CAD build for the part. Positions are in the model's coordinates, mm. Face numbers are marked on the shaded views. A direction names the side the tool comes from. Round coordinates to 2 decimals unless told otherwise and drop trailing zeros. Loops run counter-clockwise (first coordinate to the right, second up) from the corner with the lowest first, then second, coordinate; pieces in that order, holes last. Notation, with made-up numbers: M -26.75,55.5 L 27.25,55.5 A16 cw 27.25,76.5 Z; hole C 22.25,87.5 d6. An arc over 180 degrees is marked long. Use a Markdown table: item, result. Add a question column.
(1) Band-saw the part on D-D, the plane y = -55. Write the cut outline in (x, z).
(2) Wall check: L1, parallel to Y at x = 0, z = 219; L2, parallel to Z at x = -27, y = 82.5; L3, parallel to X at y = -53, z = 37. Give the ranges that are in metal, low to high.
(3) Band-saw the part on A-A, the plane x = 0. Write the cut outline in (y, z), and give its area (3 significant figures).
(4) Flat gauge pins, fed straight in: P1, Ø1, axis at x = -11, y = -79.5, coming from the +Z side; P2, Ø22, axis at x = -0.5, y = 1.5, coming from the +Z side; P3, Ø11, axis at x = 1, z = 12, coming from the +Y side; P4, Ø6, axis at y = -55, z = 16.5, coming from the +X side. Where does each tip first touch, or does it go through?
(5) Which spindle directions (+Z, -Z, +X, -X, +Y, -Y) get a long thin tool onto all of the face, cutting with end or side? Do the marked faces 1, 2 and 3. Say none if no direction does.
(6) Band-saw the part on C-C, the plane z = 157. Write the cut outline in (x, y), and give its area (3 significant figures).
from build123d import *

# Parameters (mm, degrees)
SKETCH1_R           = 47.5
BOSS_EXTRUDE1_DEPTH = 230
SKETCH2_R           = 10
CUT_EXTRUDE1_DEPTH  = 20
SKETCH3_R           = 100
BOSS_EXTRUDE2_DEPTH = 10
RIB1_REACH          = 272
SKETCH4_WALL_W      = 601.63430221
SKETCH4_WALL_H      = 10
CIRPATTERN1_COUNT   = 4
SKETCH7_OUTSIDE_W   = 276.188
SKETCH7_OUTSIDE_H   = 276.188
SKETCH7_OUTSIDE_W_2 = 135
SKETCH7_OUTSIDE_H_2 = 135
CUT_EXTRUDE2_DEPTH  = 73


with BuildPart() as part:
    # Sketch1 → Boss-Extrude1 (new body)
    with BuildSketch(Plane.XY):
        Circle(SKETCH1_R)
    extrude(amount=BOSS_EXTRUDE1_DEPTH)

    # Sketch2 → Cut-Extrude1 (cut)
    with BuildSketch(Plane.XY.offset(230)):
        Circle(SKETCH2_R)
    extrude(amount=-CUT_EXTRUDE1_DEPTH, mode=Mode.SUBTRACT)

    # Sketch3 → Boss-Extrude2 (add)
    with BuildSketch(Plane(origin=(0, 0, 0), x_dir=(-1, 0, 0), z_dir=(0, 0, -1))):
        Circle(SKETCH3_R)
    extrude(amount=BOSS_EXTRUDE2_DEPTH)

    # Sketch4 wall → Rib1 (add, up to next)
    with BuildSketch(Plane(origin=(-63.75, 0, 25), x_dir=(-0.544988350595, 0, -0.838443616301), z_dir=(-0.838443616301, 0, 0.544988350595)), mode=Mode.PRIVATE) as rib1_sk1:
        Rectangle(SKETCH4_WALL_W, SKETCH4_WALL_H)
    rib1_tool1 = extrude(rib1_sk1.sketch, amount=-RIB1_REACH, mode=Mode.PRIVATE) - part.part
    rib1 = rib1_tool1.solids().sort_by_distance((-63.75, 0, 25))[0]
    add(rib1)

    # CirPattern1: Rib1 ×4 about axis
    cirpattern1_axis = Axis((0, 0, 0), (0, 0, 1))
    for i in range(1, CIRPATTERN1_COUNT):
        add(rib1.rotate(cirpattern1_axis, i * 360 / CIRPATTERN1_COUNT))

    # Sketch7 outside → Cut-Extrude2 (cut)
    with BuildSketch(Plane.XY):
        Rectangle(SKETCH7_OUTSIDE_W, SKETCH7_OUTSIDE_H)
        Rectangle(SKETCH7_OUTSIDE_W_2, SKETCH7_OUTSIDE_H_2, mode=Mode.SUBTRACT)
    extrude(amount=CUT_EXTRUDE2_DEPTH, mode=Mode.SUBTRACT)


solid = part.part
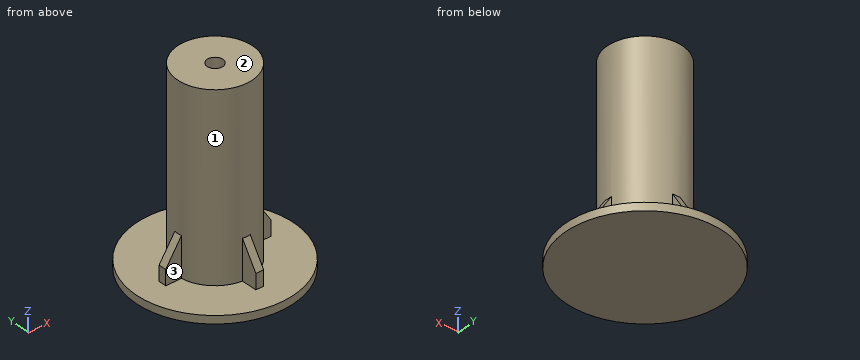
Return value:
| question | item | result |
|---|---|---|
| 1 | outline | M -83.52,-10 L 83.52,-10 L 83.52,0 L 5,0 L 5,38.46 L -5,38.46 L -5,0 L -83.52,0 Z |
| 2 | L1 | -47.5 to -10, 10 to 47.5 |
| 2 | L2 | -10 to 0 |
| 2 | L3 | -5 to 5 |
| 3 | outline | M -100,-10 L 100,-10 L 100,0 L 67.5,0 L 67.5,19.23 L 47.5,50 L 47.5,230 L 10,230 L 10,210 L -10,210 L -10,230 L -47.5,230 L -47.5,50 L -67.5,19.23 L -67.5,0 L -100,0 Z |
| 3 | area | 24,800 mm^2 |
| 4 | P1 | z = 0 |
| 4 | P2 | z = 230 |
| 4 | P3 | y = 67.5 |
| 4 | P4 | x = 5 |
| 5 | face 1 | +Z |
| 5 | face 2 | +Z, +X, -X, +Y, -Y |
| 5 | face 3 | +Z, -X, -Y |
| 6 | outline | C 0,0 d95 |
| 6 | area | 7,090 mm^2 |
